```python
from build123d import *

# Parameters (mm, degrees)
F0_W     = 13.5
F0_H     = 97
F2_DEPTH = 12
F1_W     = 13.5
F1_H     = 97
F3_DEPTH = 1.5


with BuildPart() as f2:
    # F0 (on Top) → F2 (new body)
    with BuildSketch(Plane.XY):
        Rectangle(F0_W, F0_H)
        Polygon((5.25, -46), (5.25, -47), (-5.25, -47), (-5.25, -46), (-3.25, -46), (-3.25, -45), (-5.25, -45), (-5.25, 45), (-3.25, 45), (-3.25, 46), (-5.25, 46), (-5.25, 47), (5.25, 47), (5.25, 46), (3.25, 46), (3.25, 45), (5.25, 45), (5.25, -45), (3.25, -45), (3.25, -46), align=None, mode=Mode.SUBTRACT)
    extrude(amount=F2_DEPTH)

    # F1 (on Top) → F3 (join)
    with BuildSketch(Plane.XY):
        Rectangle(F1_W, F1_H)
    extrude(amount=F3_DEPTH)


solid = f2.part
```
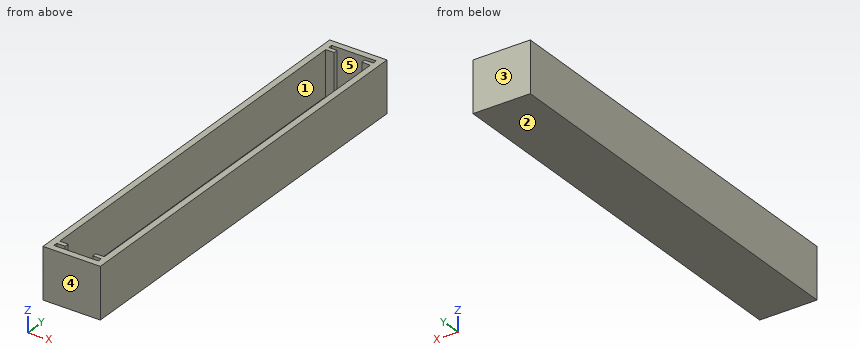
Can you work these out from the model? Positions are in its coordinate system, mm. Face numbers are marked on the shaded views. A direction names the side the tool comes from. Coordinates: 2 decimals unless noted, no trailing zeros. Loops run counter-clockwise (first coordinate to the right, second up) from the corner with the lowest first, then second, coordinate; pieces in that order, holes last. Notation, with made-up numbers: (85, -33) - (113, -33) arc R16 ccw to (113, -9) - close; hole circle Ø1 at (-35.5, -28.5). An arc over 180 degrees is marked (long way). Answer as CSV lines item,"result". Start each with the question number.
1) Suppose I cut it at B-B (z = 9.75). Please give me the cut outline in (x, y), plus the area to 4 significant figures.
2) Suppose I cut it at A-A (x = -2.25). Please give me the cut outline in (y, z), plus the area to 3 significant figures.
3) Suppose I cut it at C-C (y = 24.5). Please give me the cut outline in (x, z).
4) For pin 1 (5 mm diameter, centred on x = -2.5, y = 19.5, fed in from +Z), with a flat end and sliding along its axis, tell me the tip position at first contact or that it passes through.
5) Suppose I cut it at D-D (x = 4.25). Please give me the cut outline in (y, z).
6) I need wall thicknesses on line 1 (Y direction, x = 4.75, z = 9); line 2 (Y direction, x = -3, z = 4); line 3 (X direction, y = -27, z = 9.5). Which ranges of each line are inside material? Lowest first, please. Write a range as from..to.
7) Thinking about a two-plate mould opening in Y: for the marked faces 1, 2 and 3, which applies, pulls with the +Y half, pulls with the -Y half, needs draft (parallel to the pull), parting line crosses it, or undercut?
8) Which directions (+Z, -Z, +X, -X, +Y, -Y) give clear straight access to the entire face, cutting with the end or side of a thin tool? Please do the marked faces 4 and 5.
Check result:
1,outline,"(-6.75, -48.5) - (6.75, -48.5) - (6.75, 48.5) - (-6.75, 48.5) - close; hole (-5.25, -47) - (5.25, -47) - (5.25, -46) - (3.25, -46) - (3.25, -45) - (5.25, -45) - (5.25, 45) - (3.25, 45) - (3.25, 46) - (5.25, 46) - (5.25, 47) - (-5.25, 47) - (-5.25, 46) - (-3.25, 46) - (-3.25, 45) - (-5.25, 45) - (-5.25, -45) - (-3.25, -45) - (-3.25, -46) - (-5.25, -46) - close"
1,area,"330.5 mm²"
2,outline,"(-48.5, 0) - (48.5, 0) - (48.5, 12) - (47, 12) - (47, 1.5) - (-47, 1.5) - (-47, 12) - (-48.5, 12) - close"
2,area,"177 mm²"
3,outline,"(-6.75, 0) - (6.75, 0) - (6.75, 12) - (5.25, 12) - (5.25, 1.5) - (-5.25, 1.5) - (-5.25, 12) - (-6.75, 12) - close"
4,pin 1,"stops at z = 1.5"
5,outline,"(-48.5, 0) - (48.5, 0) - (48.5, 12) - (47, 12) - (47, 1.5) - (46, 1.5) - (46, 12) - (45, 12) - (45, 1.5) - (-45, 1.5) - (-45, 12) - (-46, 12) - (-46, 1.5) - (-47, 1.5) - (-47, 12) - (-48.5, 12) - close"
6,line 1,"y = -48.5..-47, -46..-45, 45..46, 47..48.5"
6,line 2,"y = -48.5..-47, 47..48.5"
6,line 3,"x = -6.75..-5.25, 5.25..6.75"
7,face 1,"undercut"
7,face 2,"needs draft"
7,face 3,"pulls with the +Y half"
8,face 4,"+Z, -Z, +X, -X, -Y"
8,face 5,"+Z"
